Build history of the part. All positions in model axes, mm. Round coordinates to 2 decimals unless told otherwise and drop trailing zeros. Write each loop counter-clockwise with the first axis right and the second up, starting at its lowest first coordinate (ties: lowest second). Pieces come first, ordered by that corner, then holes.
Item 1: Wall check: probe 1 along Y at (x, z) = (54, 0.55); probe 2 along X at (y, z) = (-4, 2.7); probe 3 along X at (y, z) = (34, 1.55). Give the ranges that are in metal, low to high.
Item 2: Band-saw the part on B-B, the plane y = 11. Write the cut outline in (x, z), then the cut area to 3 significant figures.
Item 3: Band-saw the part on C-C, the plane x = 21. Write the cut outline in (y, z), then the cut area to 3 significant figures.
Item 4: Band-saw the part on A-A, the plane x = 54. Write the cut outline in (y, z), then the cut area to 3 significant figures.
Item 5: Drop a flat-ended pin along its axis: pin 1 Ø3.5 at (x, y) = (54, 34) entering from +Z. Give the stop position or say it passes through.
Item 6: Band-saw the part on D-D, the plane y = -4. Write the cut outline in (x, z), then the cut area to 3 significant figures.
```python
from build123d import *

# Parameters (mm, degrees)
CYLINDER007_R     = 3
CYLINDER007_DEPTH = 3
CYLINDER006_R     = 3
CYLINDER006_DEPTH = 3
CYLINDER004_R     = 3
CYLINDER004_DEPTH = 3
CYLINDER005_R     = 3
CYLINDER005_DEPTH = 3
CYLINDER001_R     = 1.5
CYLINDER001_DEPTH = 10
CYLINDER002_R     = 1.5
CYLINDER002_DEPTH = 10
CYLINDER003_R     = 1.5
CYLINDER003_DEPTH = 10
CYLINDER_R        = 1.5
CYLINDER_DEPTH    = 10
BOX_W             = 50
BOX_H             = 30
BOX_DEPTH         = 3
BOX002_W          = 47
BOX002_H          = 27
BOX002_DEPTH      = 6
BOX001_W          = 66
BOX001_H          = 46
BOX001_DEPTH      = 3
CHAMFER_SIZE      = 2
CHAMFER001_SIZE   = 2


with BuildPart() as obj1:
    # Cylinder007 → Cylinder007 (new body)
    with BuildSketch(Plane(origin=(54, -4, -2), x_dir=(1, 0, 0), z_dir=(0, 0, 1))):
        Circle(CYLINDER007_R)
    extrude(amount=CYLINDER007_DEPTH)


with BuildPart() as obj2:
    # Cylinder006 → Cylinder006 (new body)
    with BuildSketch(Plane(origin=(54, 34, -2), x_dir=(1, 0, 0), z_dir=(0, 0, 1))):
        Circle(CYLINDER006_R)
    extrude(amount=CYLINDER006_DEPTH)


with BuildPart() as obj3:
    # Cylinder004 → Cylinder004 (new body)
    with BuildSketch(Plane(origin=(-4, -4, -2), x_dir=(1, 0, 0), z_dir=(0, 0, 1))):
        Circle(CYLINDER004_R)
    extrude(amount=CYLINDER004_DEPTH)


with BuildPart() as compound001:
    # Cylinder005 → Cylinder005 (new body)
    with BuildSketch(Plane(origin=(-4, 34, -2), x_dir=(1, 0, 0), z_dir=(0, 0, 1))):
        Circle(CYLINDER005_R)
    extrude(amount=CYLINDER005_DEPTH)

    # Compound001: union obj1, obj2, obj3
    add(obj1.part)
    add(obj2.part)
    add(obj3.part)


with BuildPart() as compound001_1:
    # Compound001 placement: moved
    add(compound001.part.moved(Location((0, 0, 4))))


with BuildPart() as obj4:
    # Cylinder001 → Cylinder001 (new body)
    with BuildSketch(Plane(origin=(54, -4, -2), x_dir=(1, 0, 0), z_dir=(0, 0, 1))):
        Circle(CYLINDER001_R)
    extrude(amount=CYLINDER001_DEPTH)


with BuildPart() as obj5:
    # Cylinder002 → Cylinder002 (new body)
    with BuildSketch(Plane(origin=(54, 34, -2), x_dir=(1, 0, 0), z_dir=(0, 0, 1))):
        Circle(CYLINDER002_R)
    extrude(amount=CYLINDER002_DEPTH)


with BuildPart() as obj6:
    # Cylinder003 → Cylinder003 (new body)
    with BuildSketch(Plane(origin=(-4, -4, -2), x_dir=(1, 0, 0), z_dir=(0, 0, 1))):
        Circle(CYLINDER003_R)
    extrude(amount=CYLINDER003_DEPTH)


with BuildPart() as compound:
    # Cylinder → Cylinder (new body)
    with BuildSketch(Plane(origin=(-4, 34, -2), x_dir=(1, 0, 0), z_dir=(0, 0, 1))):
        Circle(CYLINDER_R)
    extrude(amount=CYLINDER_DEPTH)

    # Compound: union obj4, obj5, obj6
    add(obj4.part)
    add(obj5.part)
    add(obj6.part)


with BuildPart() as krychle:
    # Box → Box (new body)
    with BuildSketch(Plane.XY.offset(0.8)):
        with Locations((25, 15)):
            Rectangle(BOX_W, BOX_H)
    extrude(amount=BOX_DEPTH)


with BuildPart() as krychle002:
    # Box002 → Box002 (new body)
    with BuildSketch(Plane(origin=(1.5, 1.5, -1), x_dir=(1, 0, 0), z_dir=(0, 0, 1))):
        with Locations((23.5, 13.5)):
            Rectangle(BOX002_W, BOX002_H)
    extrude(amount=BOX002_DEPTH)


with BuildPart() as obj7:
    # Box001 → Box001 (new body)
    with BuildSketch(Plane(origin=(-8, -8, 0), x_dir=(1, 0, 0), z_dir=(0, 0, 1))):
        with Locations((33, 23)):
            Rectangle(BOX001_W, BOX001_H)
    extrude(amount=BOX001_DEPTH)

    # Cut: cut Krychle002
    add(krychle002.part, mode=Mode.SUBTRACT)

    # Cut001: cut Krychle
    add(krychle.part, mode=Mode.SUBTRACT)

    # Cut002: cut Compound
    add(compound.part, mode=Mode.SUBTRACT)

    # Cut003: cut Compound001
    add(compound001_1.part, mode=Mode.SUBTRACT)

    # Chamfer
    chamfer_edges = [obj7.edges().sort_by_distance(p)[0] for p in [
        (-8, -8, 1.5),
        (58, -8, 1.5),
    ]]
    chamfer(chamfer_edges, length=CHAMFER_SIZE)

    # Chamfer001
    chamfer001_edges = [obj7.edges().sort_by_distance(p)[0] for p in [
        (-8, 38, 1.5),
        (58, 38, 1.5),
    ]]
    chamfer(chamfer001_edges, length=CHAMFER001_SIZE)


solid = obj7.part
```
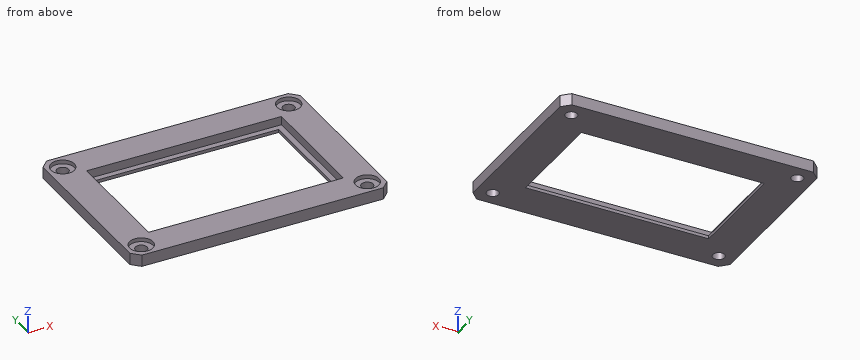
Results:
1. probe 1: y = -8 to -5.5, -2.5 to 32.5, 35.5 to 38
1. probe 2: x = -8 to -7, -1 to 51, 57 to 58
1. probe 3: x = -8 to -5.5, -2.5 to 52.5, 55.5 to 58
2. outline: (-8, 0) - (1.5, 0) - (1.5, 0.8) - (0, 0.8) - (0, 3) - (-8, 3) - close; (48.5, 0) - (58, 0) - (58, 3) - (50, 3) - (50, 0.8) - (48.5, 0.8) - close
2. area: 50.4 mm2
3. outline: (-8, 0) - (1.5, 0) - (1.5, 0.8) - (0, 0.8) - (0, 3) - (-8, 3) - close; (28.5, 0) - (38, 0) - (38, 3) - (30, 3) - (30, 0.8) - (28.5, 0.8) - close
3. area: 50.4 mm2
4. outline: (-8, 0) - (-5.5, 0) - (-5.5, 2) - (-7, 2) - (-7, 3) - (-8, 3) - close; (-2.5, 0) - (32.5, 0) - (32.5, 2) - (31, 2) - (31, 3) - (-1, 3) - (-1, 2) - (-2.5, 2) - close; (35.5, 0) - (38, 0) - (38, 3) - (37, 3) - (37, 2) - (35.5, 2) - close
4. area: 114 mm2
5. pin 1: stops at z = 2
6. outline: (-8, 0) - (-5.5, 0) - (-5.5, 2) - (-7, 2) - (-7, 3) - (-8, 3) - close; (-2.5, 0) - (52.5, 0) - (52.5, 2) - (51, 2) - (51, 3) - (-1, 3) - (-1, 2) - (-2.5, 2) - close; (55.5, 0) - (58, 0) - (58, 3) - (57, 3) - (57, 2) - (55.5, 2) - close
6. area: 174 mm2
